from build123d import *

# Parameters (mm, degrees)
SKETCH1_R           = 1.4605
BOSS_EXTRUDE1_DEPTH = 5.9944


with BuildPart() as part:
    # Sketch1 → Boss-Extrude1 (new body)
    with BuildSketch(Plane.XY):
        with BuildLine():
            Line((4.6355, 0), (4.6355, 0.4445))
            ThreePointArc((4.6355, 0.4445), (5.007474388, 1.342525612), (5.9055, 1.7145))
            Line((5.9055, 1.7145), (6.35, 1.7145))
            ThreePointArc((6.35, 1.7145), (10.9855, 6.35), (6.35, 10.9855))
            Line((6.35, 10.9855), (5.9055, 10.9855))
            ThreePointArc((5.9055, 10.9855), (5.007474388, 11.357474388), (4.6355, 12.2555))
            Line((4.6355, 12.2555), (4.6355, 57.15))
            ThreePointArc((4.6355, 57.15), (0, 61.7855), (-4.6355, 57.15))
            Line((-4.6355, 57.15), (-4.6355, 0))
            ThreePointArc((-4.6355, 0), (0, -4.6355), (4.6355, 0))
        make_face()
        Circle(SKETCH1_R, mode=Mode.SUBTRACT)
        with Locations((0, 6.35)):
            Circle(SKETCH1_R, mode=Mode.SUBTRACT)
        with Locations((6.35, 6.35)):
            Circle(SKETCH1_R, mode=Mode.SUBTRACT)
    extrude(amount=BOSS_EXTRUDE1_DEPTH)


solid = part.part
Geometry: final body of the model. Coordinates: model frame, mm. A direction names the side the tool comes from. Coordinates: 2 decimals unless noted, no trailing zeros. Order: outer loops, then holes, each group sorted by start corner. A loop starts at its lowest first (then second) coordinate and runs counter-clockwise, first axis right, second up. Notation, with made-up numbers: (6, 71.5) - (22, 71.5) arc R26 ccw to (22, 103.5) - close; hole circle Ø3 at (36, 8.25). An arc over 180 degrees is marked (long way). Use one line per item in the form item = value.
1) Section A-A (x = 0). Return loops of the section in (y, z), then the cut area to 3 significant figures.
Solutions:
outline = (-4.64, 0) - (-1.46, 0) - (-1.46, 5.99) - (-4.64, 5.99) - close; (1.46, 0) - (4.89, 0) - (4.89, 5.99) - (1.46, 5.99) - close; (7.81, 0) - (61.79, 0) - (61.79, 5.99) - (7.81, 5.99) - close
area = 363 mm^2
2) Set-up query: faces 1 (the face through (4.636, 34, 3)), 2 (the face through (0, 29, 0)). Return all of +Z, -Z, +X, -X, +Y, -Y with unobstructed straight access to the full face (end or side cutting, diameter ignored); none if empty.
Solutions:
face_1 = +Z, -Z, +X, +Y
face_2 = -Z, +X, -X, +Y, -Y
3) Section C-C (z = 4.05). Return loops of the section in (x, y), then the cut area to 3 significant figures.
Solutions:
outline = (-4.64, 0) arc R4.64 ccw to (4.64, 0) - (4.64, 0.44) arc R1.27 cw to (5.91, 1.71) - (6.35, 1.71) arc R4.64 ccw to (6.35, 10.99) - (5.91, 10.99) arc R1.27 cw to (4.64, 12.26) - (4.64, 57.15) arc R4.64 ccw to (-4.64, 57.15) - close; hole circle Ø2.92 at (0, 0); hole circle Ø2.92 at (0, 6.35); hole circle Ø2.92 at (6.35, 6.35)
area = 628 mm^2
4) Ray query, L1, parallel to Y at x = 0, z = 4.5; L2, parallel to Y at x = -0.75, z = 1.9; L3, parallel to Y at x = 6.35, z = 2.65. Return the intervals inside material, ascending.
Solutions:
L1 = -4.64 to -1.46, 1.46 to 4.89, 7.81 to 61.79
L2 = -4.57 to -1.25, 1.25 to 5.1, 7.6 to 61.72
L3 = 1.71 to 4.89, 7.81 to 10.99
5) Section D-D (y = 14). Return loops of the section in (x, z).
Solutions:
outline = (-4.64, 0) - (4.64, 0) - (4.64, 5.99) - (-4.64, 5.99) - close
6) Section B-B (y = 6.35). Return loops of the section in (x, z), then the cut area to 3 significant figures.
Solutions:
outline = (-4.64, 0) - (-1.46, 0) - (-1.46, 5.99) - (-4.64, 5.99) - close; (1.46, 0) - (4.89, 0) - (4.89, 5.99) - (1.46, 5.99) - close; (7.81, 0) - (10.99, 0) - (10.99, 5.99) - (7.81, 5.99) - close
area = 58.6 mm^2
7) Pin query (flat end, axial travel): pin 1 (0.5 mm diameter, centred on y = 0.5, z = 3.5, fed in from +X); pin 2 (0.5 mm diameter, centred on x = 6, z = 3, fed in from -Y). Return the tip coordinate at first contact, or that it passes through.
Solutions:
pin_1 = 4.67
pin_2 = 1.7
